Geometry: final body of the model. Coordinates: model frame, mm. A direction names the side the tool comes from. Round coordinates to 2 decimals unless told otherwise and drop trailing zeros. Write each loop counter-clockwise with the first axis right and the second up, starting at its lowest first coordinate (ties: lowest second). Pieces come first, ordered by that corner, then holes. Notation, with made-up numbers: (25.5, 60) - (38.5, 60) arc R30 ccw to (38.5, 98) - close; hole circle Ø1 at (-11, -16.5). An arc over 180 degrees is marked (long way). Write each question's results on one line, items separated by ' | '.
from build123d import *

# Parameters (mm, degrees)
SKETCH1_R           = 5
BOSS_EXTRUDE1_DEPTH = 43
BOSS_EXTRUDE2_DEPTH = 6.4
FILLET1_R           = 1


with BuildPart() as part:
    # Sketch1 → Boss-Extrude1 (new body)
    with BuildSketch(Plane(origin=(0, 0, 0), x_dir=(1, 0, 0), z_dir=(0, 1, 0))):
        with Locations(Location((0, 0, 0), (0, 0, 270))):
            Circle(SKETCH1_R)
    extrude(amount=BOSS_EXTRUDE1_DEPTH)

    # Sketch2 → Boss-Extrude2 (add)
    with BuildSketch(Plane.XZ):
        Polygon((4.907477288, 8.5), (-4.907477288, 8.5), (-9.814954576, 0), (-4.907477288, -8.5), (4.907477288, -8.5), (9.814954576, 0), align=None)
    extrude(amount=BOSS_EXTRUDE2_DEPTH)

    # Fillet1
    fillet1_edges = [part.edges().sort_by_distance(p)[0] for p in [
        (0, 0, -5),
    ]]
    fillet(fillet1_edges, radius=FILLET1_R)


solid = part.part
Q1. Ray query, line 1 along Y through (x, z) = (4, 4.75); line 2 along X through (y, z) = (10.5, -2); line 3 along X through (y, z) = (26.5, -1). Return the intervals inside material, ascending.
Answer block:
line 1: -6.4 to 0 | line 2: -4.58 to 4.58 | line 3: -4.9 to 4.9
Q2. Section query A-A, the plane x = 0. Return loops of the section in (y, z), plus the area to 3 significant figures.
Answer block:
outline: (-6.4, -8.5) - (0, -8.5) - (0, -6) arc R1 cw to (1, -5) - (43, -5) - (43, 5) - (1, 5) arc R1 cw to (0, 6) - (0, 8.5) - (-6.4, 8.5) - close | area: 539 mm2
Q3. Section query B-B, the plane y = -2. Return loops of the section in (x, z).
Answer block:
outline: (-9.81, 0) - (-4.91, -8.5) - (4.91, -8.5) - (9.81, 0) - (4.91, 8.5) - (-4.91, 8.5) - close
Q4. Pin query (flat end, axial travel): pin 1 (4 mm diameter, centred on x = 4.5, y = 33, fed in from -Z); pin 2 (8 mm diameter, centred on y = 2, z = -4, fed in from +X); pin 3 (6 mm diameter, centred on y = 26.5, z = 5, fed in from -X). Return the tip coordinate at first contact, or that it passes through.
Answer block:
pin 1: z = -4.33 | pin 2: x = 9.51 | pin 3: x = -4.58
Q5. Access query for faces 1 (the cylindrical face through (-4.88, 21.71, -1.08)), 2 (the flat face through (7.396, -3.155, 4.191)). Directions: +Z, -Z, +X, -X, +Y, -Y. A direction counts if a zero-diameter tool reaches every point of the face in a straight line with its end or side. Return the directions, or none.
Answer block:
face 1: +Y | face 2: +Z, +X, +Y, -Y
Q6. Section query C-C, the plane z = 7. Return loops of the section in (x, y), plus the area to 3 significant figures.
Answer block:
outline: (-5.77, -6.4) - (5.77, -6.4) - (5.77, 0) - (-5.77, 0) - close | area: 73.9 mm2
Q7. Section query D-D, the plane y = 40. Return loops of the section in (x, z), plus the area to 3 significant figures.
Answer block:
outline: circle Ø10 at (0, 0) | area: 78.5 mm2
